Geometry check sheet. Reference: drawing and pictorial views, mm from the part's lowest x, y, z. A direction names the side the tool comes from. Round coordinates to 2 decimals unless told otherwise and drop trailing zeros. Loops run counter-clockwise (first coordinate to the right, second up) from the corner with the lowest first, then second, coordinate; pieces in that order, holes last. Notation, with made-up numbers: (-15, 85.5) - (0, 85.5) arc R32 cw to (0, 116.5) - close; hole circle Ø10 at (9, -21). An arc over 180 degrees is marked (long way). Answer in a Markdown table with one row per item. Add a question column.
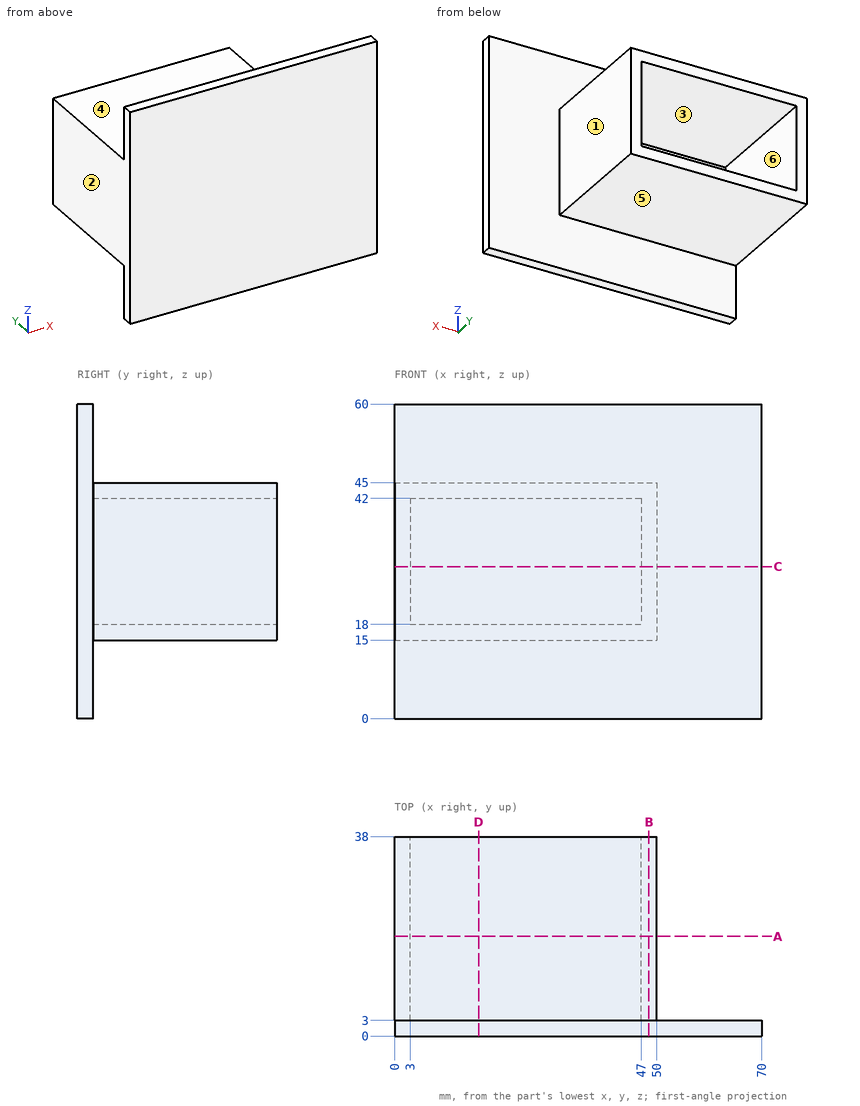
Q1. Scan lines: line 1 (Z direction, x = 42.5, y = 32); line 2 (X direction, y = 10, z = 30.5); line 3 (Y direction, x = 54, z = 24.5). Record each from-to range of solid material in increasing order. Write a range as from..to.
Q2. Cross-section at A-A, the plane y = 19. Enter the section's corners in (x, z), plus the area to 3 significant figures.
Q3. Depth check by flat-ended pin: P1, Ø3, axis at x = 52, z = 48, coming from the +Y side; P2, Ø9, axis at y = 18, z = 26, coming from the +X side; P3, Ø1.5, axis at x = 49.5, y = 18.5, coming from the -Z side. Enter the tip coordinate at first touch or a pass-through.
Q4. Cross-section at C-C, the plane z = 29. Enter the section's corners in (x, y).
Q5. Cross-section at B-B, the plane x = 48.5. Enter the section's corners in (y, z), plus the area to 3 significant figures.
Q6. Set-up check for the marked faces 1 and 2: record each of +Z, -Z, +X, -X, +Y, -Y from which the full face is reachable in a straight line by a thin tool's end or side.
Q7. Cross-section at D-D, the plane x = 16. Enter the section's corners in (y, z).
Q8. Release check for a two-part mould opening along Z. For the marked faces 3, 4, 5 and 6 record: +Z half, -Z half, draft (parallel to the pull), parting line (faces both ways), or undercut.
Check sheet entries:
| question | item | result |
|---|---|---|
| 1 | line 1 | 15..18, 42..45 |
| 1 | line 2 | 0..3, 47..50 |
| 1 | line 3 | 0..3 |
| 2 | outline | (0, 15) - (50, 15) - (50, 45) - (0, 45) - close; hole (3, 18) - (47, 18) - (47, 42) - (3, 42) - close |
| 2 | area | 444 mm² |
| 3 | P1 | y = 3 |
| 3 | P2 | x = 50 |
| 3 | P3 | z = 15 |
| 4 | outline | (0, 0) - (70, 0) - (70, 3) - (50, 3) - (50, 38) - (47, 38) - (47, 3) - (3, 3) - (3, 38) - (0, 38) - close |
| 5 | outline | (0, 0) - (3, 0) - (3, 15) - (38, 15) - (38, 45) - (3, 45) - (3, 60) - (0, 60) - close |
| 5 | area | 1,230 mm² |
| 6 | face 1 | +Z, -Z, +X, +Y |
| 6 | face 2 | +Z, -Z, -X, +Y, -Y |
| 7 | outline | (0, 0) - (3, 0) - (3, 15) - (38, 15) - (38, 18) - (3, 18) - (3, 42) - (38, 42) - (38, 45) - (3, 45) - (3, 60) - (0, 60) - close |
| 8 | face 3 | undercut |
| 8 | face 4 | +Z half |
| 8 | face 5 | -Z half |
| 8 | face 6 | undercut |
